The model under review builds one solid part; all positions refer to its coordinate system, in mm. Face numbers are marked on the shaded views. Give positions to 0.01 mm unless a question says otherwise; leave off trailing zeros. Loops run counter-clockwise (first coordinate to the right, second up) from the corner with the lowest first, then second, coordinate; pieces in that order, holes last. Notation, with made-up numbers: (17, 28.25) -> (44, 28.25) arc R16 ccw to (44, 52.25) -> close; hole circle Ø1 at (63, 6.5). An arc over 180 degrees is marked (long way). Write each question's results on one line, items separated by ' | '. Start each with the question number.
Q1. We need section A-A (y = 43.5). Write out the cut boundary in (x, z).
Q2. Mouldability with a two-part tool opening along X and no side actions: class the marked faces 1, 2, 3 and 4 as released by +X, released by -X, zero draft, split by the parting line, or undercut.
Q3. Insertion check: pin 1 Ø4 at (x, y) = (-5.5, 49.5) entering from +Z; pin 2 Ø6.5 at (x, z) = (2.5, 4.5) entering from +Y; pin 3 Ø12 at (y, z) = (23.5, -3) entering from -X. Each pin has a flat end and moves straight along its axis. Give the tip position at first contact, or say it passes through.
Q4. Wall thickness on L1, parallel to X at y = 57, z = 0.5; L2, parallel to Y at x = 3.5, z = 1.5; L3, parallel to Y at x = -9.5, z = -3.75: over which ranges is each line inside the solid? List them lowest first. Write a range as [from, to].
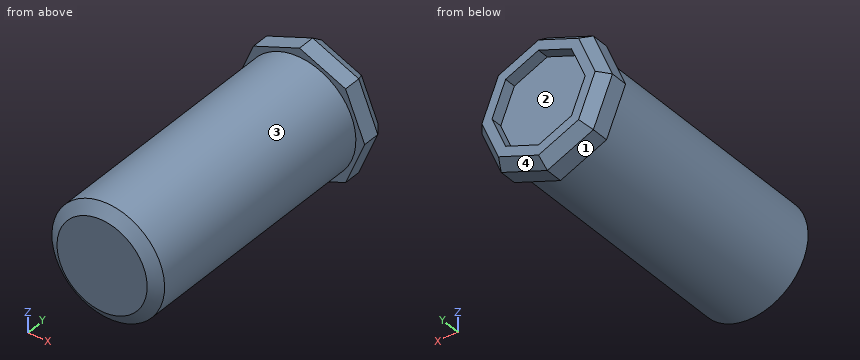
from build123d import *
from OCP.BRepFilletAPI import BRepFilletAPI_MakeChamfer

# Parameters (mm, degrees)
SKETCH1_R           = 12.7
BOSS_EXTRUDE1_DEPTH = 57.15
BOSS_EXTRUDE2_DEPTH = 6.35
CHAMFER1_SIZE       = 2.54
CHAMFER1_SIZE2      = 1.778527147
CUT_EXTRUDE1_DEPTH  = 2.54
CHAMFER2_SIZE       = 2.54
CHAMFER2_SIZE2      = 1.778527147


with BuildPart() as part:
    # Sketch1 → Boss-Extrude1 (new body)
    with BuildSketch(Plane(origin=(0, 0, 0), x_dir=(1, 0, 0), z_dir=(0, 1, 0))):
        with Locations(Location((0, 0, 0), (0, 0, 270))):
            Circle(SKETCH1_R)
    extrude(amount=BOSS_EXTRUDE1_DEPTH)

    # Sketch2 → Boss-Extrude2 (add)
    with BuildSketch(Plane(origin=(0, 57.15, 0), x_dir=(1, 0, 0), z_dir=(0, 1, 0))):
        Polygon((0, 14.681421742), (-10.381332871, 10.381332871), (-14.681421742, 0), (-10.381332871, -10.381332871), (0, -14.681421742), (10.381332871, -10.381332871), (14.681421742, 0), (10.381332871, 10.381332871), align=None)
    extrude(amount=BOSS_EXTRUDE2_DEPTH)

    # Chamfer1: one chamfer whose edges measure the first distance from different faces: ONE call of the kernel's chamfer builder (chamfer() names one face for all edges)
    chamfer1_edges_1 = [part.edges().sort_by_distance(p)[0] for p in [
        (5.190666436, 63.5, 12.531377306),
    ]]
    chamfer1_side_1 = [part.faces().sort_by_distance(p)[0] for p in [
        (5.190666436, 60.325, 12.531377306),
    ]]
    chamfer1_edges_2 = [part.edges().sort_by_distance(p)[0] for p in [
        (12.531377306, 63.5, 5.190666436),
    ]]
    chamfer1_side_2 = [part.faces().sort_by_distance(p)[0] for p in [
        (12.531377306, 60.325, 5.190666436),
    ]]
    chamfer1_edges_3 = [part.edges().sort_by_distance(p)[0] for p in [
        (12.531377306, 63.5, -5.190666436),
    ]]
    chamfer1_side_3 = [part.faces().sort_by_distance(p)[0] for p in [
        (12.531377306, 60.325, -5.190666436),
    ]]
    chamfer1_edges_4 = [part.edges().sort_by_distance(p)[0] for p in [
        (5.190666436, 63.5, -12.531377306),
    ]]
    chamfer1_side_4 = [part.faces().sort_by_distance(p)[0] for p in [
        (5.190666436, 60.325, -12.531377306),
    ]]
    chamfer1_edges_5 = [part.edges().sort_by_distance(p)[0] for p in [
        (-5.190666436, 63.5, -12.531377306),
    ]]
    chamfer1_side_5 = [part.faces().sort_by_distance(p)[0] for p in [
        (-5.190666436, 60.325, -12.531377306),
    ]]
    chamfer1_edges_6 = [part.edges().sort_by_distance(p)[0] for p in [
        (-12.531377306, 63.5, -5.190666436),
    ]]
    chamfer1_side_6 = [part.faces().sort_by_distance(p)[0] for p in [
        (-12.531377306, 60.325, -5.190666436),
    ]]
    chamfer1_edges_7 = [part.edges().sort_by_distance(p)[0] for p in [
        (-12.531377306, 63.5, 5.190666436),
    ]]
    chamfer1_side_7 = [part.faces().sort_by_distance(p)[0] for p in [
        (-12.531377306, 60.325, 5.190666436),
    ]]
    chamfer1_edges_8 = [part.edges().sort_by_distance(p)[0] for p in [
        (-5.190666436, 63.5, 12.531377306),
    ]]
    chamfer1_side_8 = [part.faces().sort_by_distance(p)[0] for p in [
        (-5.190666436, 60.325, 12.531377306),
    ]]
    chamfer1 = BRepFilletAPI_MakeChamfer(part.part.solid().wrapped)
    for e in chamfer1_edges_1:
        chamfer1.Add(CHAMFER1_SIZE, CHAMFER1_SIZE2, e.wrapped, chamfer1_side_1[0].wrapped)  # the first distance lies on this face
    for e in chamfer1_edges_2:
        chamfer1.Add(CHAMFER1_SIZE, CHAMFER1_SIZE2, e.wrapped, chamfer1_side_2[0].wrapped)  # the first distance lies on this face
    for e in chamfer1_edges_3:
        chamfer1.Add(CHAMFER1_SIZE, CHAMFER1_SIZE2, e.wrapped, chamfer1_side_3[0].wrapped)  # the first distance lies on this face
    for e in chamfer1_edges_4:
        chamfer1.Add(CHAMFER1_SIZE, CHAMFER1_SIZE2, e.wrapped, chamfer1_side_4[0].wrapped)  # the first distance lies on this face
    for e in chamfer1_edges_5:
        chamfer1.Add(CHAMFER1_SIZE, CHAMFER1_SIZE2, e.wrapped, chamfer1_side_5[0].wrapped)  # the first distance lies on this face
    for e in chamfer1_edges_6:
        chamfer1.Add(CHAMFER1_SIZE, CHAMFER1_SIZE2, e.wrapped, chamfer1_side_6[0].wrapped)  # the first distance lies on this face
    for e in chamfer1_edges_7:
        chamfer1.Add(CHAMFER1_SIZE, CHAMFER1_SIZE2, e.wrapped, chamfer1_side_7[0].wrapped)  # the first distance lies on this face
    for e in chamfer1_edges_8:
        chamfer1.Add(CHAMFER1_SIZE, CHAMFER1_SIZE2, e.wrapped, chamfer1_side_8[0].wrapped)  # the first distance lies on this face
    add(Compound.cast(chamfer1.Shape()), mode=Mode.REPLACE)

    # Sketch3 → Cut-Extrude1 (cut)
    with BuildSketch(Plane(origin=(0, 63.5, 0), x_dir=(1, 0, 0), z_dir=(0, 1, 0))):
        Polygon((0, 10.493107574), (-7.419747521, 7.419747521), (-10.493107574, 0), (-7.419747521, -7.419747521), (0, -10.493107574), (7.419747521, -7.419747521), (10.493107574, 0), (7.419747521, 7.419747521), align=None)
    extrude(amount=-CUT_EXTRUDE1_DEPTH, mode=Mode.SUBTRACT)

    # Chamfer2
    chamfer2_edges = [part.edges().sort_by_distance(p)[0] for p in [
        (0, 0, -12.7),
    ]]
    chamfer2_side = [part.faces().sort_by_distance(p)[0] for p in [
        (0, 0, 0),
    ]]
    chamfer(chamfer2_edges, length=CHAMFER2_SIZE, length2=CHAMFER2_SIZE2, reference=chamfer2_side[0])


solid = part.part
Output:
1) outline: circle Ø25.4 at (0, 0)
2) face 1: released by -X | face 2: undercut | face 3: split by the parting line | face 4: released by +X
3) pin 1: z = 12.21 | pin 2: y = 60.96 | pin 3: x = -12.7
4) L1: [-12.69, 12.69] | L2: [0, 60.96] | L3: [0.04, 63.5]
